Part model, mm, in its own coordinate system. Give positions to 0.01 mm unless a question says otherwise; leave off trailing zeros. Loops run counter-clockwise (first coordinate to the right, second up) from the corner with the lowest first, then second, coordinate; pieces in that order, holes last. Notation, with made-up numbers: (48, 32) -> (66, 32) arc R26 cw to (66, 63) -> close; hole circle Ø9 at (15.5, 60.5). An arc over 180 degrees is marked (long way). Write item = value, one per line.
from build123d import *

# Parameters (mm, degrees)
SKETCH2_R = 0.4


with BuildPart() as part:
    # Sweep1: sweep along a path in Sketch1
    with BuildLine(Plane(origin=(0, 0, 0), x_dir=(0, 0, -1), z_dir=(1, 0, 0))) as sweep1_path:
        Line((2.76, 4.177906174), (2.76, -4.177906174))
        ThreePointArc((2.76, -4.177906174), (2.689503998, -4.433887259), (2.497894737, -4.617685771))
        ThreePointArc((2.497894737, -4.617685771), (0, -5.25), (-2.497894737, -4.617685771))
        ThreePointArc((-2.497894737, -4.617685771), (-2.689503998, -4.433887259), (-2.76, -4.177906174))
        Line((-2.76, -4.177906174), (-2.76, 4.177906174))
        ThreePointArc((-2.76, 4.177906174), (-2.689503998, 4.433887259), (-2.497894737, 4.617685771))
        ThreePointArc((-2.497894737, 4.617685771), (0, 5.25), (2.497894737, 4.617685771))
        ThreePointArc((2.497894737, 4.617685771), (2.689503998, 4.433887259), (2.76, 4.177906174))
    # Sketch2 → Sweep1 (sweep)
    with BuildSketch(Plane(origin=(0, 0, 0), x_dir=(1, 0, 0), z_dir=(0, 1, 0))):
        with Locations((0, 3.26)):
            Circle(SKETCH2_R)
    sweep(path=sweep1_path.line)


solid = part.part
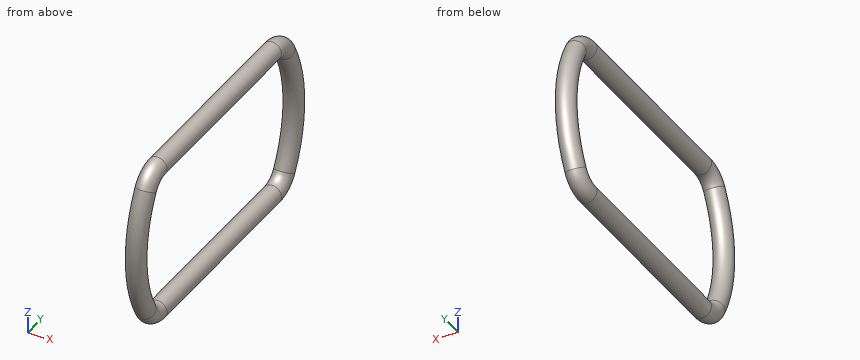
1) Slice it at B-B, the plane y = -3.25. List the corners of the cut face in (x, z).
Resolved:
outline = circle Ø0.8 at (0, -3.26); circle Ø0.8 at (0, 3.26)
2) Drill centre lines: line 1 along Z through (x, y) = (-0.05, 2); line 2 along Z through (x, y) = (-0.1, 2); line 3 along Y through (x, z) = (-0.3, 2). Where is each one in solid material? Low to high. Write a range as [from, to].
Resolved:
line_1 = [-3.66, -2.86], [2.86, 3.66]
line_2 = [-3.65, -2.87], [2.87, 3.65]
line_3 = [-5.67, -5.11], [5.11, 5.67]
3) Drop a flat-ended pin along its axis: P1, Ø1, axis at y = 3.5, z = 2, coming from the +X side. Give the stop position or say it passes through.
Resolved:
P1 = through
4) Slice it at A-A, the plane x = 0. List the corners of the cut face in (y, z), and give its area (3 significant figures).
Resolved:
outline = (-5.41, -2.93) arc R1.4 ccw to (-4.18, -3.66) -> (4.18, -3.66) arc R1.4 ccw to (5.41, -2.93) arc R6.15 ccw to (5.41, 2.93) arc R1.4 ccw to (4.18, 3.66) -> (-4.18, 3.66) arc R1.4 ccw to (-5.41, 2.93) arc R6.15 ccw to start; hole (-4.71, -2.55) arc R0.6 ccw to (-4.18, -2.86) -> (4.18, -2.86) arc R0.6 ccw to (4.71, -2.55) arc R5.35 ccw to (4.71, 2.55) arc R0.6 ccw to (4.18, 2.86) -> (-4.18, 2.86) arc R0.6 ccw to (-4.71, 2.55) arc R5.35 ccw to start
area = 25.9 mm²
